```python
from build123d import *

# Parameters (mm, degrees)
F0_R     = 14.2875
F0_R_2   = 3.175
F1_DEPTH = 6.35


with BuildPart() as f1:
    # F0 (on Front) → F1 (new body)
    with BuildSketch(Plane.XZ):
        with BuildLine():
            Line((-6.35, -63.5), (0, -63.5))
            Line((0, -63.5), (50.8, -63.5))
            Line((50.8, -63.5), (57.15, -63.5))
            ThreePointArc((57.15, -63.5), (61.640128, -61.640128), (63.5, -57.15))
            Line((63.5, -57.15), (63.5, -44.45))
            ThreePointArc((63.5, -44.45), (61.640128, -39.959872), (57.15, -38.1))
            ThreePointArc((57.15, -38.1), (52.659872, -36.240128), (50.8, -31.75))
            Line((50.8, -31.75), (50.8, -25.4))
            ThreePointArc((50.8, -25.4), (43.360512, -7.439488), (25.4, 0))
            ThreePointArc((25.4, 0), (7.439488, -7.439488), (0, -25.4))
            Line((0, -25.4), (0, -31.75))
            ThreePointArc((0, -31.75), (-1.859872, -36.240128), (-6.35, -38.1))
            ThreePointArc((-6.35, -38.1), (-10.840128, -39.959872), (-12.7, -44.45))
            Line((-12.7, -44.45), (-12.7, -57.15))
            ThreePointArc((-12.7, -57.15), (-10.840128, -61.640128), (-6.35, -63.5))
        make_face()
        with Locations((25.4, -25.4)):
            Circle(F0_R, mode=Mode.SUBTRACT)
        with BuildLine():
            Line((50.8, -63.5), (0, -63.5))
            Line((0, -63.5), (-6.35, -63.5))
            ThreePointArc((-6.35, -63.5), (-10.840128, -61.640128), (-12.7, -57.15))
            Line((-12.7, -57.15), (-12.7, -76.2))
            ThreePointArc((-12.7, -76.2), (-10.840128, -80.690128), (-6.35, -82.55))
            Line((-6.35, -82.55), (57.15, -82.55))
            ThreePointArc((57.15, -82.55), (61.640128, -80.690128), (63.5, -76.2))
            Line((63.5, -76.2), (63.5, -57.15))
            ThreePointArc((63.5, -57.15), (61.640128, -61.640128), (57.15, -63.5))
            Line((57.15, -63.5), (50.8, -63.5))
        make_face()
        with Locations((-6.35, -76.2)):
            Circle(F0_R_2, mode=Mode.SUBTRACT)
        with Locations((57.15, -76.2)):
            Circle(F0_R_2, mode=Mode.SUBTRACT)
    extrude(amount=F1_DEPTH)


solid = f1.part
```
Geometry: final body of the model. Coordinates: model frame, mm. A direction names the side the tool comes from. Round coordinates to 2 decimals unless told otherwise and drop trailing zeros. Loops run counter-clockwise (first coordinate to the right, second up) from the corner with the lowest first, then second, coordinate; pieces in that order, holes last. Notation, with made-up numbers: (62, -35) -> (70, -35) arc R17 cw to (70, -31) -> close; hole circle Ø1 at (-12, 7). An arc over 180 degrees is marked (long way). Use one line per item in the form item = value.
Item 1: Material intervals for probe 1 along X at (y, z) = (-1, -79); probe 2 along Z at (x, y) = (-6.35, -1.75) (3 decimals); probe 3 along X at (y, z) = (-3, -78), sorted ascending.
Evaluation:
probe_1 = -12.05 to -7.85, -4.85 to 55.65, 58.65 to 62.85
probe_2 = -82.55 to -79.375, -73.025 to -38.1
probe_3 = -12.44 to -8.97, -3.73 to 54.53, 59.77 to 63.24
Item 2: Access query for faces 1 (the flat face through (25, 0, -50)), 2 (the flat face through (0, -3, -29)), 3 (the flat face through (50.8, -3, -29)). Directions: +Z, -Z, +X, -X, +Y, -Y. A direction counts if a zero-diameter tool reaches every point of the face in a straight line with its end or side. Return the directions, or none.
Evaluation:
face_1 = +Z, -Z, +X, -X, +Y
face_2 = +Z, -X, +Y, -Y
face_3 = +Z, +X, +Y, -Y
Item 3: Cut plane A-A on y = -3.25. Give the number of separate pieces and of enclosed holes in the cut face, then the cut area to 3 significant figures.
Evaluation:
separate_pieces = 1
enclosed_holes = 3
area = 4,320 mm2
Item 4: Cut plane B-B on z = -74. Output: boundary loops of the cut face in (x, y), then the cut area to 3 significant figures.
Evaluation:
outline = (-12.7, -6.35) -> (-8.64, -6.35) -> (-8.64, 0) -> (-12.7, 0) -> close; (-4.06, -6.35) -> (54.86, -6.35) -> (54.86, 0) -> (-4.06, 0) -> close; (59.44, -6.35) -> (63.5, -6.35) -> (63.5, 0) -> (59.44, 0) -> close
area = 426 mm2
Item 5: Cut plane C-C on x = 33.5. Output: boundary loops of the cut face in (y, z).
Evaluation:
outline = (-6.35, -82.55) -> (0, -82.55) -> (0, -37.17) -> (-6.35, -37.17) -> close; (-6.35, -13.63) -> (0, -13.63) -> (0, -1.33) -> (-6.35, -1.33) -> close
Item 6: Cut plane D-D on x = 2. Output: boundary loops of the cut face in (y, z).
Evaluation:
outline = (-6.35, -82.55) -> (0, -82.55) -> (0, -15.52) -> (-6.35, -15.52) -> close
Item 7: Contact query for flat-ended pins moving along their axis: pin 1 Ø1.5 at (x, y) = (10, -2.5) entering from +Z; pin 2 Ø4 at (x, z) = (-1, -13.5) entering from +Y; pin 3 Ø3 at (y, z) = (-3.5, -27.5) entering from +X. Output: stop coordinate, or through.
Evaluation:
pin_1 = -4.65
pin_2 = through
pin_3 = 50.8
Item 8: Draft query along Z for faces 4 (the cylindrical face through (14.87, -3.131, -15.744)), 5 (the cylindrical face through (61.59, -3.13, -80.74)), 6 (the flat face through (63.5, -3, -61)). Return one class per face: released by +Z, released by -Z, zero draft, split by the parting line, or undercut.
Evaluation:
face_4 = undercut
face_5 = released by -Z
face_6 = zero draft
